from build123d import *

# Parameters (mm, degrees)
F0_R     = 3.25
F1_DEPTH = 4


with BuildPart() as f1:
    # F0 (on Top) → F1 (new body)
    with BuildSketch(Plane.XY):
        Circle(F0_R)
        with BuildLine():
            ThreePointArc((2.1999961154, 0.4717171738), (2.2374641069, 0.2371800374), (2.25, 0))
            ThreePointArc((2.25, 0), (2.2374641069, -0.2371800374), (2.1999961154, -0.4717171738))
            ThreePointArc((2.1999961154, -0.4717171738), (2.5256218299, -0.7287723318), (2.6485571585, -1.125))
            ThreePointArc((2.6485571585, -1.125), (2.2501959894, -1.7566755621), (1.5085171137, -1.6693939373))
            ThreePointArc((1.5085171137, -1.6693939373), (1.125, -1.9485571585), (0.6914790018, -2.1411111111))
            ThreePointArc((0.6914790018, -2.1411111111), (0.6978664991, -2.1953891093), (0.7, -2.25))
            ThreePointArc((0.7, -2.25), (-0.0546108907, -2.9478664991), (-0.6914790018, -2.1411111111))
            ThreePointArc((-0.6914790018, -2.1411111111), (-1.125, -1.9485571585), (-1.5085171137, -1.6693939373))
            ThreePointArc((-1.5085171137, -1.6693939373), (-2.5547749412, -1.475), (-2.1999961154, -0.4717171738))
            ThreePointArc((-2.1999961154, -0.4717171738), (-2.25, 0), (-2.1999961154, 0.4717171738))
            ThreePointArc((-2.1999961154, 0.4717171738), (-2.5547749412, 1.475), (-1.5085171137, 1.6693939373))
            ThreePointArc((-1.5085171137, 1.6693939373), (-1.125, 1.9485571585), (-0.6914790018, 2.1411111111))
            ThreePointArc((-0.6914790018, 2.1411111111), (-0.0546108907, 2.9478664991), (0.7, 2.25))
            ThreePointArc((0.7, 2.25), (0.6978664991, 2.1953891093), (0.6914790018, 2.1411111111))
            ThreePointArc((0.6914790018, 2.1411111111), (1.125, 1.9485571585), (1.5085171137, 1.6693939373))
            ThreePointArc((1.5085171137, 1.6693939373), (2.2501959894, 1.7566755621), (2.6485571585, 1.125))
            ThreePointArc((2.6485571585, 1.125), (2.5256218299, 0.7287723318), (2.1999961154, 0.4717171738))
        make_face(mode=Mode.SUBTRACT)
        with BuildLine():
            ThreePointArc((1.5085171137, 1.6693939373), (1.9485571585, 1.125), (2.1999961154, 0.4717171738))
            ThreePointArc((2.1999961154, 0.4717171738), (2.5256218299, 0.7287723318), (2.6485571585, 1.125))
            ThreePointArc((2.6485571585, 1.125), (2.2501959894, 1.7566755621), (1.5085171137, 1.6693939373))
        make_face()
        with BuildLine():
            ThreePointArc((2.6485571585, -1.125), (2.5256218299, -0.7287723318), (2.1999961154, -0.4717171738))
            ThreePointArc((2.1999961154, -0.4717171738), (1.9485571585, -1.125), (1.5085171137, -1.6693939373))
            ThreePointArc((1.5085171137, -1.6693939373), (2.2501959894, -1.7566755621), (2.6485571585, -1.125))
        make_face()
        with BuildLine():
            ThreePointArc((-0.6914790018, 2.1411111111), (0, 2.25), (0.6914790018, 2.1411111111))
            ThreePointArc((0.6914790018, 2.1411111111), (0.6978664991, 2.1953891093), (0.7, 2.25))
            ThreePointArc((0.7, 2.25), (-0.0546108907, 2.9478664991), (-0.6914790018, 2.1411111111))
        make_face()
        with BuildLine():
            ThreePointArc((0.7, -2.25), (0.6978664991, -2.1953891093), (0.6914790018, -2.1411111111))
            ThreePointArc((0.6914790018, -2.1411111111), (0, -2.25), (-0.6914790018, -2.1411111111))
            ThreePointArc((-0.6914790018, -2.1411111111), (-0.0546108907, -2.9478664991), (0.7, -2.25))
        make_face()
        with BuildLine():
            ThreePointArc((-2.1999961154, 0.4717171738), (-1.9485571585, 1.125), (-1.5085171137, 1.6693939373))
            ThreePointArc((-1.5085171137, 1.6693939373), (-2.5547749412, 1.475), (-2.1999961154, 0.4717171738))
        make_face()
        with BuildLine():
            ThreePointArc((-2.1999961154, -0.4717171738), (-2.5547749412, -1.475), (-1.5085171137, -1.6693939373))
            ThreePointArc((-1.5085171137, -1.6693939373), (-1.9485571585, -1.125), (-2.1999961154, -0.4717171738))
        make_face()
        with BuildLine():
            ThreePointArc((1.5085171137, 1.6693939373), (1.3423393759, 0.775), (2.1999961154, 0.4717171738))
            ThreePointArc((2.1999961154, 0.4717171738), (1.9485571585, 1.125), (1.5085171137, 1.6693939373))
        make_face()
        with BuildLine():
            ThreePointArc((1.5085171137, -1.6693939373), (1.9485571585, -1.125), (2.1999961154, -0.4717171738))
            ThreePointArc((2.1999961154, -0.4717171738), (1.3423393759, -0.775), (1.5085171137, -1.6693939373))
        make_face()
        with BuildLine():
            ThreePointArc((-0.6914790018, 2.1411111111), (0, 1.55), (0.6914790018, 2.1411111111))
            ThreePointArc((0.6914790018, 2.1411111111), (0, 2.25), (-0.6914790018, 2.1411111111))
        make_face()
        with BuildLine():
            ThreePointArc((-0.6914790018, -2.1411111111), (0, -2.25), (0.6914790018, -2.1411111111))
            ThreePointArc((0.6914790018, -2.1411111111), (0, -1.55), (-0.6914790018, -2.1411111111))
        make_face()
        with BuildLine():
            ThreePointArc((-1.2485571585, 1.125), (-1.3168815965, 1.4266388309), (-1.5085171137, 1.6693939373))
            ThreePointArc((-1.5085171137, 1.6693939373), (-1.9485571585, 1.125), (-2.1999961154, 0.4717171738))
            ThreePointArc((-2.1999961154, 0.4717171738), (-1.5523294903, 0.5479353287), (-1.2485571585, 1.125))
        make_face()
        with BuildLine():
            ThreePointArc((-2.1999961154, -0.4717171738), (-1.9485571585, -1.125), (-1.5085171137, -1.6693939373))
            ThreePointArc((-1.5085171137, -1.6693939373), (-1.3168815965, -1.4266388309), (-1.2485571585, -1.125))
            ThreePointArc((-1.2485571585, -1.125), (-1.5523294903, -0.5479353287), (-2.1999961154, -0.4717171738))
        make_face()
    extrude(amount=F1_DEPTH)


solid = f1.part
Check sheet for the modelled part. Datum: model origin and axes. Units: mm. Coordinates: 2 decimals unless noted, no trailing zeros. Loops run counter-clockwise (first coordinate to the right, second up) from the corner with the lowest first, then second, coordinate; pieces in that order, holes last. Notation, with made-up numbers: (72, 35) -> (112, 35) arc R22 ccw to (112, 69) -> close; hole circle Ø7 at (19, 12). An arc over 180 degrees is marked (long way). Write item = value, one per line. Start each with the question number.
1. Section check C-C on z = 1.05. Record the cut outline in (x, y) (3 decimals), then the cut area to 3 significant figures.
2. Section check A-A on x = 0. Record the cut outline in (y, z).
3. Section check B-B on y = 2. Record the cut outline in (x, z).
4. Depth check by flat-ended pin: P1, Ø2, axis at y = 1.5, z = 3, coming from the -X side; P2, Ø2, axis at x = -1.5, y = -2.5, coming from the -Z side; P3, Ø1.5, axis at x = 2.5, z = 3, coming from the +Y side. Enter the tip coordinate at first touch or a pass-through.
5. Section check D-D on y = -0.75. Record the cut outline in (x, z).
6. Draft check along X on faces 1 (the cylindrical face through (-2.25, -0.01, 1.97)), 2 (the cylindrical face through (-2.579, -1.978, 1.972)), 3 (the cylindrical face through (1.35, -0.76, 1.97)), 4 (the flat face through (-1.5, -1.4, 4)). Enter one of: released by +X, released by -X, zero draft, split by the parting line, or undercut.
7. Material ranges on line 1 (Y direction, x = 0, z = 1.4); line 2 (X direction, y = 1.75, z = 3.7); line 3 (Y direction, x = 2, z = 2.5), recorded low to high.
Responses:
q1.outline = circle Ø6.5 at (0, 0); hole (-2.2, -0.472) arc R0.7 cw to (-1.509, -1.669) arc R2.25 ccw to (-0.691, -2.141) arc R0.7 cw to (0.691, -2.141) arc R2.25 ccw to (1.509, -1.669) arc R0.7 cw to (2.2, -0.472) arc R2.25 ccw to (2.2, 0.472) arc R0.7 cw to (1.509, 1.669) arc R2.25 ccw to (0.691, 2.141) arc R0.7 cw to (-0.691, 2.141) arc R2.25 ccw to (-1.509, 1.669) arc R0.7 cw to (-2.2, 0.472) arc R2.25 ccw to start
q1.area = 21.6 mm2
q2.outline = (-3.25, 0) -> (-1.55, 0) -> (-1.55, 4) -> (-3.25, 4) -> close; (1.55, 0) -> (3.25, 0) -> (3.25, 4) -> (1.55, 4) -> close
q3.outline = (-2.56, 0) -> (-1.03, 0) -> (-1.03, 4) -> (-2.56, 4) -> close; (-0.65, 0) -> (0.65, 0) -> (0.65, 4) -> (-0.65, 4) -> close; (1.03, 0) -> (2.56, 0) -> (2.56, 4) -> (1.03, 4) -> close
q4.P1 = -3.21
q4.P2 = 0
q4.P3 = 2.74
q5.outline = (-3.16, 0) -> (-1.36, 0) -> (-1.36, 4) -> (-3.16, 4) -> close; (1.36, 0) -> (3.16, 0) -> (3.16, 4) -> (1.36, 4) -> close
q6.face_1 = undercut
q6.face_2 = split by the parting line
q6.face_3 = undercut
q6.face_4 = zero draft
q7.line_1 = -3.25 to -1.55, 1.55 to 3.25
q7.line_2 = -2.74 to -1.41, -0.49 to 0.49, 1.41 to 2.74
q7.line_3 = -2.56 to -0.43, 0.43 to 2.56
